```python
from build123d import *

# Parameters (mm, degrees)
F0_W          = 41
F0_H          = 28.5
F0_R          = 1.5
F1_DEPTH      = 1
F3_DEPTH      = 5
F3_DEPTH_BACK = 5
F4_R          = 0.5
F5_DEPTH      = 6


with BuildPart() as f1:
    # F0 (on Top) → F1 (new body)
    with BuildSketch(Plane.XY):
        Rectangle(F0_W, F0_H)
        with Locations((-18, -11.75)):
            Circle(F0_R, mode=Mode.SUBTRACT)
        with Locations((18, -11.75)):
            Circle(F0_R, mode=Mode.SUBTRACT)
        with Locations((-18, 11.75)):
            Circle(F0_R, mode=Mode.SUBTRACT)
        with Locations((18, 11.75)):
            Circle(F0_R, mode=Mode.SUBTRACT)
    extrude(amount=F1_DEPTH)

    # F2 (on Right) → F3 (join, two sides)
    with BuildSketch(Plane.YZ) as f3_sk:
        Polygon((-13.774308, 0.989061), (-12.100797, 0.989061), (-12.100797, 4.378995), (-16.49913, 4.378995), (-16.49913, 2.147646), (-13.774308, 2.147646), align=None)
    extrude(amount=F3_DEPTH)
    extrude(f3_sk.sketch, amount=-F3_DEPTH_BACK)

    # F4 (on face) → F5 (join)
    with BuildSketch(Plane.XZ.offset(16.49913)):
        with Locations((-4.071627, 3.263321)):
            Circle(F4_R)
        with Locations((-1.571627, 3.263321)):
            Circle(F4_R)
        with Locations((0.928373, 3.263321)):
            Circle(F4_R)
        with Locations((3.428373, 3.263321)):
            Circle(F4_R)
    extrude(amount=F5_DEPTH)


solid = f1.part
```
Can you work these out from the model? Positions are in its coordinate system, mm. A direction names the side the tool comes from. Round coordinates to 2 decimals unless told otherwise and drop trailing zeros. Loops run counter-clockwise (first coordinate to the right, second up) from the corner with the lowest first, then second, coordinate; pieces in that order, holes last. Notation, with made-up numbers: M 22,-15 L 40,-15 A26 ccw 40,7 Z; hole C 77,67 d5. An arc over 180 degrees is marked long. Answer as a JSON object with one key per item and string values. Group by question number.
Q1. Imagine slicing it at A-A, the plane y = 11.75. Please give me the cut outline in (x, z).
Q2. Imagine slicing it at C-C, the plane x = -11. Please give me the cut outline in (y, z), then the cut area to 3 significant figures.
Q3. Will these pins go through, and if not, where does the flat tip stop? pin 1 (0.9 mm diameter, centred on x = 1.5, z = 1.5, fed in from -Y); pin 2 (2.5 mm diameter, centred on x = -18, y = 11.75, fed in from -Z); pin 3 (1 mm diameter, centred on x = -2, z = 3.5, fed in from +Y); pin 4 (1.7 mm diameter, centred on y = -15, z = 3, fed in from -X).
Q4. Imagine slicing it at B-B, the plane x = -18. Please give me the cut outline in (y, z), then the cut area to 3 significant figures.
Q5. On a 3-axis mill with a long thin cutter (end or side, diameter ignored), from which of +Z, -Z, +X, -X, +Y, -Y can I reach the whole of each face in a straight line? I mean faces 4 (the cylindrical face through (16.5, -11.7, 0.5)), 5 (the flat face through (-5, -14, 3)), 6 (the flat face through (0.1, -13.774, 1.6)), 7 (the cylindrical face through (-1.68, -19.457, 2.775)). Say none if no direction works.
Q6. Imagine slicing it at D-D, the plane y = 0.5. Please give me the cut outline in (x, z), then the cut area to 3 significant figures.
Q7. Please list where these lines run through material, in increasing order: L1, parallel to Y at x = -18, z = 0.7; L2, parallel to Z at x = 3, y = -11; L3, parallel to Y at x = 10.5, z = 0.35.
Q8. We'd pull the mould along X, two halves only. Please class faces 1 (the cylindrical face through (-19.5, -11.7, 0.5)), 2 (the flat face through (-20.5, -0.2, 0.5)), 3 (the flat face through (0, 0, 0)): +X half, -X half, draft (parallel to the pull), parting line (faces both ways), or undercut.
Findings:
{
 "1": {"outline": "M -20.5,0 L -19.5,0 L -19.5,1 L -20.5,1 Z; M -16.5,0 L 16.5,0 L 16.5,1 L -16.5,1 Z; M 19.5,0 L 20.5,0 L 20.5,1 L 19.5,1 Z"},
 "2": {"outline": "M -14.25,0 L 14.25,0 L 14.25,1 L -14.25,1 Z", "area": "28.5 mm2"},
 "3": {"pin 1": "stops at y = -13.77", "pin 2": "passes through", "pin 3": "stops at y = -12.1", "pin 4": "stops at x = -5"},
 "4": {"outline": "M -14.25,0 L -13.25,0 L -13.25,1 L -14.25,1 Z; M -10.25,0 L 10.25,0 L 10.25,1 L -10.25,1 Z; M 13.25,0 L 14.25,0 L 14.25,1 L 13.25,1 Z", "area": "22.5 mm2"},
 "5": {"face 4": "+Z, -Z", "face 5": "+Z, -X, +Y, -Y", "face 6": "+X, -X, -Y", "face 7": "-Y"},
 "6": {"outline": "M -20.5,0 L 20.5,0 L 20.5,1 L -20.5,1 Z", "area": "41.0 mm2"},
 "7": {"L1": "y = -14.25 to -13.25, -10.25 to 10.25, 13.25 to 14.25", "L2": "z = 0 to 1", "L3": "y = -14.25 to 14.25"},
 "8": {"face 1": "undercut", "face 2": "-X half", "face 3": "draft"}
}
